Build history of the part. All positions in model axes, mm. Face numbers are marked on the shaded views. A direction names the side the tool comes from. Coordinates: 2 decimals unless noted, no trailing zeros. Order: outer loops, then holes, each group sorted by start corner. A loop starts at its lowest first (then second) coordinate and runs counter-clockwise, first axis right, second up. Notation, with made-up numbers: (64, 53.5) - (121, 53.5) arc R26 cw to (121, 84.5) - close; hole circle Ø5 at (67, -23). An arc over 180 degrees is marked (long way). Answer as CSV lines item,"result". Start each with the question number.
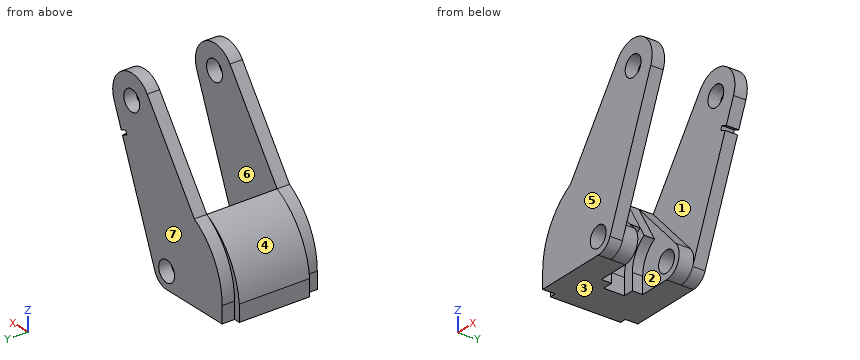
from build123d import *
from build123d.topology import SkipClean

# Parameters (mm, degrees)
SKETCH2_R           = 5
BOSS_EXTRUDE1_DEPTH = 6
BOSS_EXTRUDE2_START = 7
SKETCH3_R           = 5
BOSS_EXTRUDE2_DEPTH = 7
BOSS_EXTRUDE3_START = 5
SKETCH4_W           = 22.995704609
SKETCH4_H           = 8
BOSS_EXTRUDE3_DEPTH = 5
BOSS_EXTRUDE4_START = 5
SKETCH5_W           = 18
SKETCH5_H           = 8
BOSS_EXTRUDE4_DEPTH = 5
MIRROR1_START       = -40
MIRROR1_OUTLINE_R   = 5
MIRROR1_DEPTH       = 6
MIRROR1_START_2     = -34
MIRROR1_2_DEPTH     = 17
MIRROR1_3_OUTLINE_R = 5
MIRROR1_3_DEPTH     = 7
MIRROR1_START_3     = -27
MIRROR1_4_DEPTH     = 5
CUT_EXTRUDE1_DEPTH  = 14


# Read off the part's stored shape, not the designer's step: Mirror1
with BuildPart() as part:
    # Sketch2 → Boss-Extrude1 (new body)
    with BuildSketch(Plane(origin=(0, 0, 0), x_dir=(1, 0, 0), z_dir=(0, 1, 0))):
        with BuildLine():
            ThreePointArc((7.415342239, 3.002115835), (4.471189625, 6.633887498), (0, 8))
            Line((0, 8), (-35, 8))
            Line((-35, 8), (-35, 0))
            ThreePointArc((-35, 0), (-30.310889132, -17.5), (-17.5, -30.310889132))
            Line((-17.5, -30.310889132), (12.232451358, -71.97101094))
            ThreePointArc((12.232451358, -71.97101094), (27.776984485, -75.517910927), (33.123013358, -60.496826248))
            Line((33.123013358, -60.496826248), (7.415342239, 3.002115835))
        make_face()
        with Locations(Location((0, 0, 0), (0, 0, 270))):
            Circle(SKETCH2_R, mode=Mode.SUBTRACT)
        with Locations(Location((22, -65, 0), (0, 0, 270))):
            Circle(SKETCH2_R, mode=Mode.SUBTRACT)
    extrude(amount=BOSS_EXTRUDE1_DEPTH)

    # Sketch3 → Boss-Extrude2 (add)
    with SkipClean():  # the faces are left unmerged after this step: merging them gives an invalid solid
        with BuildSketch(Plane.XZ.offset(BOSS_EXTRUDE2_START)):
            with BuildLine():
                Line((5.830508196, 5.47769789), (-17.5, 30.310889132))
                ThreePointArc((-17.5, 30.310889132), (-31.638718646, 17.785480653), (-38, 0))
                Line((-38, 0), (-38, -8))
                Line((-38, -8), (-35, -8))
                Line((-35, -8), (0, -8))
                ThreePointArc((0, -8), (7.342396854, -3.176351435), (5.830508196, 5.47769789))
            make_face()
            with Locations(Location((0, 0, 0), (0, 0, 270))):
                Circle(SKETCH3_R, mode=Mode.SUBTRACT)
        extrude(amount=-BOSS_EXTRUDE2_DEPTH)

    # Sketch4 → Boss-Extrude3 (add)
    with SkipClean():  # the faces are left unmerged after this step: merging them gives an invalid solid
        with BuildSketch(Plane.XZ.offset(7).offset(BOSS_EXTRUDE3_START)):
            with BuildLine():
                Line((-38, 0), (-15.004295391, 0))
                ThreePointArc((-15.004295391, 0), (-12.994100974, 7.502147695), (-7.502147695, 12.994100974))
                Line((-7.502147695, 12.994100974), (-17.5, 30.310889132))
                ThreePointArc((-17.5, 30.310889132), (-31.638718646, 17.785480653), (-38, 0))
            make_face()
            with Locations((-26.502147695, -4)):
                Rectangle(SKETCH4_W, SKETCH4_H)
        extrude(amount=-BOSS_EXTRUDE3_DEPTH)

    # Sketch5 → Boss-Extrude4 (add)
    with SkipClean():  # the faces are left unmerged after this step: merging them gives an invalid solid
        with BuildSketch(Plane.XZ.offset(12).offset(BOSS_EXTRUDE4_START)):
            with Locations((-29, -4)):
                Rectangle(SKETCH5_W, SKETCH5_H)
            with BuildLine():
                ThreePointArc((-20, 0), (-17.320508076, 10), (-10, 17.320508076))
                Line((-10, 17.320508076), (-17.5, 30.310889132))
                ThreePointArc((-17.5, 30.310889132), (-31.638718646, 17.785480653), (-38, 0))
                Line((-38, 0), (-20, 0))
            make_face()
        extrude(amount=-BOSS_EXTRUDE4_DEPTH)



with BuildPart() as body_2:
    # Mirror1 outline → Mirror1 (new body)
    with BuildSketch(Plane(origin=(0, 0, 0), x_dir=(1, 0, 0), z_dir=(0, 1, 0)).offset(MIRROR1_START)):
        with BuildLine():
            Line((0, 8), (-35, 8))
            Line((-35, 8), (-35, 0))
            ThreePointArc((-35, 0), (-30.310889132, -17.5), (-17.5, -30.310889132))
            Line((-17.5, -30.310889132), (12.232451358, -71.97101094))
            ThreePointArc((12.232451358, -71.97101094), (27.776984485, -75.517910927), (33.123013358, -60.496826248))
            Line((33.123013358, -60.496826248), (7.415342239, 3.002115835))
            ThreePointArc((7.415342239, 3.002115835), (4.471189625, 6.633887498), (0, 8))
        make_face()
        Circle(MIRROR1_OUTLINE_R, mode=Mode.SUBTRACT)
        with Locations((22, -65)):
            Circle(MIRROR1_OUTLINE_R, mode=Mode.SUBTRACT)
    extrude(amount=MIRROR1_DEPTH)


with BuildPart() as part_1:
    with SkipClean():  # the faces are left unmerged after this step: merging them gives an invalid solid
        add(part.part)

        add(body_2.part)  # Mirror1 2 merges body 2
        # Mirror1 2 outline → Mirror1 2 (add)
        with BuildSketch(Plane(origin=(0, 0, 0), x_dir=(1, 0, 0), z_dir=(0, 1, 0)).offset(MIRROR1_START_2)):
            with BuildLine():
                ThreePointArc((-38, 0), (-31.638718646, -17.785480653), (-17.5, -30.310889132))
                Line((-17.5, -30.310889132), (-10, -17.320508076))
                ThreePointArc((-10, -17.320508076), (-17.320508076, -10), (-20, 0))
                Line((-20, 0), (-20, 8))
                Line((-20, 8), (-38, 8))
                Line((-38, 8), (-38, 0))
            make_face()
        extrude(amount=MIRROR1_2_DEPTH)

    # Mirror1 3 outline → Mirror1 3 (add)
    with SkipClean():  # the faces are left unmerged after this step: merging them gives an invalid solid
        with BuildSketch(Plane(origin=(0, 0, 0), x_dir=(1, 0, 0), z_dir=(0, 1, 0)).offset(MIRROR1_START_2)):
            with BuildLine():
                Line((-17.5, -30.310889132), (5.830508196, -5.47769789))
                ThreePointArc((5.830508196, -5.47769789), (7.342396854, 3.176351435), (0, 8))
                Line((0, 8), (-20, 8))
                Line((-20, 8), (-20, 0))
                ThreePointArc((-20, 0), (-17.320508076, -10), (-10, -17.320508076))
                Line((-10, -17.320508076), (-17.5, -30.310889132))
            make_face()
            Circle(MIRROR1_3_OUTLINE_R, mode=Mode.SUBTRACT)
        extrude(amount=MIRROR1_3_DEPTH)

    # Mirror1 4 outline → Mirror1 4 (add)
    with SkipClean():  # the faces are left unmerged after this step: merging them gives an invalid solid
        with BuildSketch(Plane(origin=(0, 0, 0), x_dir=(1, 0, 0), z_dir=(0, 1, 0)).offset(MIRROR1_START_3)):
            with BuildLine():
                ThreePointArc((-20, 0), (-17.320508076, -10), (-10, -17.320508076))
                Line((-10, -17.320508076), (-7.502147695, -12.994100974))
                ThreePointArc((-7.502147695, -12.994100974), (-12.994100974, -7.502147695), (-15.004295391, 0))
                Line((-15.004295391, 0), (-15.004295391, 8))
                Line((-15.004295391, 8), (-20, 8))
                Line((-20, 8), (-20, 0))
            make_face()
        extrude(amount=MIRROR1_4_DEPTH)

    # Sketch6 → Cut-Extrude1 (cut)
    with SkipClean():  # the faces are left unmerged after this step: merging them gives an invalid solid
        with BuildSketch(Plane(origin=(0, 6, 0), x_dir=(1, 0, 0), z_dir=(0, 1, 0))):
            Polygon((25.839086267, -50.499606328), (28.619839606, -49.37381289), (27.869310647, -47.519977331), (25.088557308, -48.645770769), align=None)
        extrude(amount=-CUT_EXTRUDE1_DEPTH, mode=Mode.SUBTRACT)


solid = part_1.part
(1) Drop flat-ended pins along their axis: pin 1 Ø2 at (x, y) = (-25.5, -22.5) entering from +Z; pin 2 Ø3 at (y, z) = (-14, 13) entering from +X (3 decimals); pin 3 Ø13 at (x, z) = (22, 65) entering from +Y; pin 4 Ø4 at (y, z) = (-9.5, -4.5) entering from +X. Give the stop position or say it passes through.
(2) Band-saw the part on C-C on y = -4.5. List the corners of the cut face in (x, z), plus the area to 3 significant figures.
(3) Pull direction Y, two halves, no side cores. Call the marked faces 4, 5, 6 and 7: +Y half, -Y half, draft (parallel to the pull), parting line (faces both ways), or undercut.
(4) Which spindle directions (+Z, -Z, +X, -X, +Y, -Y) get a long thin tool onto all of the face, cutting with end or side? Do the marked faces 1, 2 and 3. Say none if no direction does.
(5) Probe L1, parallel to X at y = -1.75, z = 0; L2, parallel to Y at x = 20.5, z = 73; L3, parallel to Y at x = -14, z = 25.5. List the from-to ranges inside material, lowest first. Write a range as [from, to].
(6) Band-saw the part on A-A on z = 65. List the corners of the cut face in (x, y), plus the area to 3 significant figures.
(7) Band-saw the part on B-B on x = 22. List the corners of the cut face in (y, z), plus the area to 3 significant figures.
(8) Band-saw the part on D-D on z = 39. List the corners of the cut face in (x, y).
Filled in:
1,pin 1,"stops at z = 25.68"
1,pin 2,"stops at x = -13.775"
1,pin 3,"stops at y = 6"
1,pin 4,"stops at x = -15"
2,outline,"(-38, -8) - (0, -8) arc R8 ccw to (5.83, 5.48) - (-17.5, 30.31) arc R38 ccw to (-38, 0) - close; hole circle Ø10 at (0, 0)"
2,area,"1,130 mm^2"
3,face 4,"draft"
3,face 5,"-Y half"
3,face 6,"undercut"
3,face 7,"+Y half"
4,face 1,"+Z, +X"
4,face 2,"+X"
4,face 3,"-Z, +X, -X, +Y, -Y"
5,L1,"x = [-38, -5], [5, 8]"
5,L2,"y = [-40, -34], [0, 6]"
5,L3,"y = [-40, -27], [-7, 6]"
6,outline,"(7.26, -40) - (17, -40) - (17, -34) - (7.26, -34) - close; (7.26, 0) - (17, 0) - (17, 6) - (7.26, 6) - close; (27, -40) - (34, -40) - (34, -34) - (27, -34) - close; (27, 0) - (34, 0) - (34, 6) - (27, 6) - close"
6,area,"201 mm^2"
7,outline,"(-40, 33.02) - (-34, 33.02) - (-34, 60) - (-40, 60) - close; (-40, 70) - (-34, 70) - (-34, 77) - (-40, 77) - close; (0, 33.02) - (6, 33.02) - (6, 60) - (0, 60) - close; (0, 70) - (6, 70) - (6, 77) - (0, 77) - close"
7,area,"408 mm^2"
8,outline,"(-11.3, -40) - (24.42, -40) - (24.42, -34) - (-11.3, -34) - close; (-11.3, 0) - (24.42, 0) - (24.42, 6) - (-11.3, 6) - close"
